Print and shaded views of the part. All mm, measured from the part's lowest x, y and z. A direction names the side the tool comes from. Round coordinates to 2 decimals unless told otherwise and drop trailing zeros. Loops run counter-clockwise (first coordinate to the right, second up) from the corner with the lowest first, then second, coordinate; pieces in that order, holes last. Notation, with made-up numbers: (-6.75, 87.25) - (5.25, 87.25) arc R36 ccw to (5.25, 123.25) - close; hole circle Ø11 at (-25.75, 7.25). An arc over 180 degrees is marked (long way). Use one line per item in the form item = value.
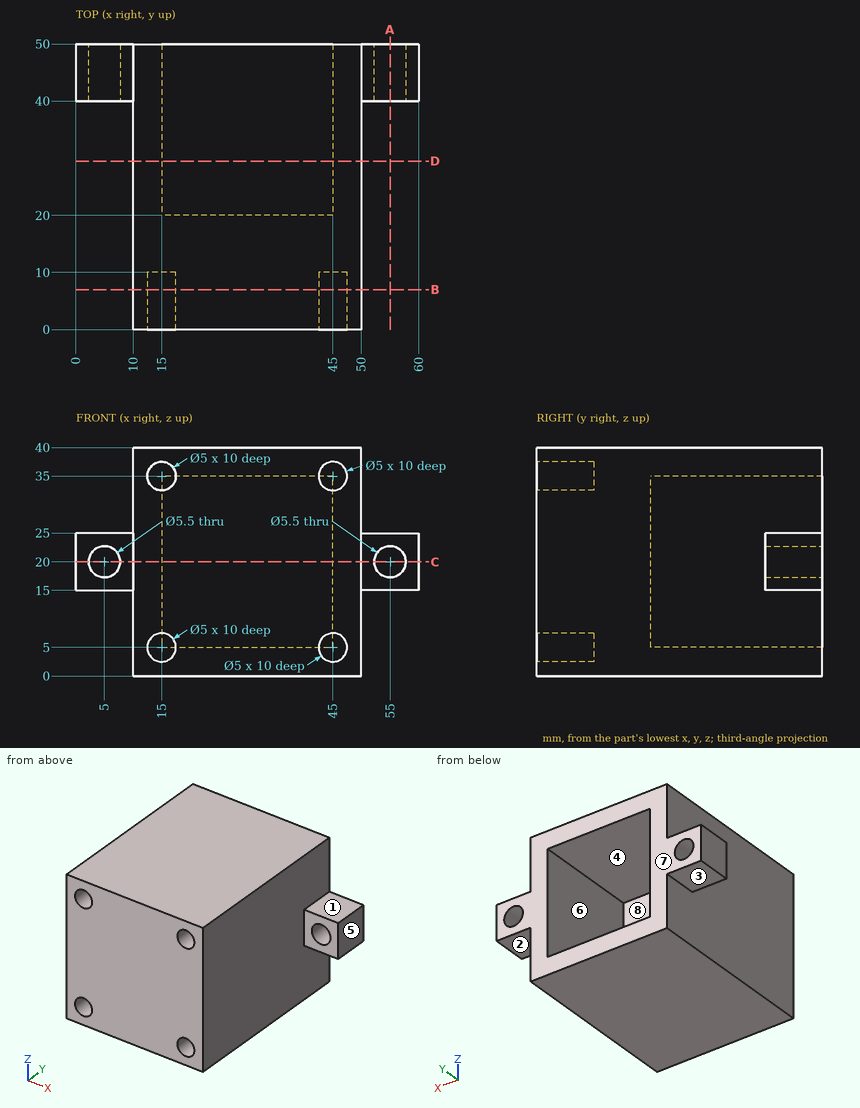
1. Cut at D-D, the plane y = 29.5. Give the cut face in (x, z), plus the area to 3 significant figures.
Geometry check:
outline = (10, 0) - (50, 0) - (50, 40) - (10, 40) - close; hole (15, 5) - (45, 5) - (45, 35) - (15, 35) - close
area = 700 mm^2
2. Flat gauge pins, fed straight in: pin 1 (10 mm diameter, centred on y = 10, z = 9, fed in from -X); pin 2 (1.5 mm diameter, centred on y = 27.5, z = 21.5, fed in from +X); pin 3 (8 mm diameter, centred on x = 57.5, y = 42.5, fed in from +Z); pin 4 (1 mm diameter, centred on x = 51, z = 30.5, fed in from -Y). Where does each tip first touch, or does it go through?
Geometry check:
pin_1 = 10
pin_2 = 50
pin_3 = 25
pin_4 = through
3. Tool access for the marked faces 1, 2, 3 and 4: list every direction of +Z, -Z, +X, -X, +Y, -Y with a clear straight run to the whole face (end or side of a thin tool).
Geometry check:
face_1 = +Z, +X, +Y, -Y
face_2 = -Z, +X, +Y, -Y
face_3 = -Z, -X, +Y, -Y
face_4 = +Y
4. Cut at C-C, the plane z = 20. Give the cut face in (x, y), plus the area to 3 significant figures.
Geometry check:
outline = (0, 40) - (2.25, 40) - (2.25, 50) - (0, 50) - close; (7.75, 40) - (10, 40) - (10, 0) - (50, 0) - (50, 40) - (52.25, 40) - (52.25, 50) - (45, 50) - (45, 20) - (15, 20) - (15, 50) - (7.75, 50) - close; (57.75, 40) - (60, 40) - (60, 50) - (57.75, 50) - close
area = 1,190 mm^2
5. Cut at A-A, the plane x = 55. Give the cut face in (y, z).
Geometry check:
outline = (40, 15) - (50, 15) - (50, 17.25) - (40, 17.25) - close; (40, 22.75) - (50, 22.75) - (50, 25) - (40, 25) - close
6. Wall check: probe 1 along X at (y, z) = (46.5, 20); probe 2 along Z at (x, y) = (15, 7.75); probe 3 along Z at (x, y) = (18, 37.5). Give the ranges that are in metal, low to high.
Geometry check:
probe_1 = 0 to 2.25, 7.75 to 15, 45 to 52.25, 57.75 to 60
probe_2 = 0 to 2.5, 7.5 to 32.5, 37.5 to 40
probe_3 = 0 to 5, 35 to 40
7. Cut at B-B, the plane y = 7. Give the cut face in (x, z), plus the area to 3 significant figures.
Geometry check:
outline = (10, 0) - (50, 0) - (50, 40) - (10, 40) - close; hole circle Ø5 at (15, 5); hole circle Ø5 at (15, 35); hole circle Ø5 at (45, 5); hole circle Ø5 at (45, 35)
area = 1,520 mm^2
8. Pull direction X, two halves, no side cores. Call the marked faces 5, 6, 7 and 8: +X half, -X half, draft (parallel to the pull), parting line (faces both ways), or undercut.
Geometry check:
face_5 = +X half
face_6 = undercut
face_7 = draft
face_8 = undercut
